```python
from build123d import *

# Parameters (mm, degrees)
F1_DEPTH = 3


with BuildPart() as f1:
    # F0 (on Front) → F1 (new body)
    with BuildSketch(Plane.XZ):
        Polygon((22.4, 25.4), (-25.4, 25.4), (-25.4, -22.4), (-12.7, -22.4), (-12.7, -25.4), (-6.35, -25.4), (-6.35, -22.4), (-1.7526, -22.4), (-1.7526, -18.650325), (-3.96875, -18.650325), (-3.96875, -15.8722), (-1.7526, -15.8722), (-1.7526, -12.6972), (1.7526, -12.6972), (1.7526, -15.8722), (3.96875, -15.8722), (3.96875, -18.650325), (1.7526, -18.650325), (1.7526, -22.4), (6.35, -22.4), (6.35, -25.4), (12.7, -25.4), (12.7, -22.4), (22.4, -22.4), (22.4, -12.7), (25.4, -12.7), (25.4, -6.35), (22.4, -6.35), (22.4, -1.7526), (18.650325, -1.7526), (18.650325, -3.9624), (15.8722, -3.9624), (15.8722, -1.7526), (12.6972, -1.7526), (12.6972, 1.7526), (15.8722, 1.7526), (15.8722, 3.9624), (18.650325, 3.9624), (18.650325, 1.7526), (22.4, 1.7526), (22.4, 6.35), (25.4, 6.35), (25.4, 12.7), (22.4, 12.7), align=None)
    extrude(amount=F1_DEPTH)


solid = f1.part
```
Input: part model. Units: mm. Frame: model coordinates. A direction names the side the tool comes from. Coordinates: 2 decimals unless noted, no trailing zeros. Loops run counter-clockwise (first coordinate to the right, second up) from the corner with the lowest first, then second, coordinate; pieces in that order, holes last. Notation, with made-up numbers: (79.5, 59.25) - (97.5, 59.25) arc R33 ccw to (97.5, 88.25) - close; hole circle Ø4 at (27, 48.25). An arc over 180 degrees is marked (long way). Answer in a Markdown table with one row per item.
(1) Pin query (flat end, axial travel): P1, Ø0.9, axis at x = 24, y = -2, coming from the -Z side; P2, Ø1.5, axis at x = -21.5, y = -2, coming from the -Z side; P3, Ø1.5, axis at y = -1, z = -24.5, coming from the -X side. Return the tip coordinate at first contact, or that it passes through.
Model answer:
| item | result |
|---|---|
| P1 | stops at z = -12.7 |
| P2 | stops at z = -22.4 |
| P3 | stops at x = -12.7 |
(2) Mould query, pull axis X, two halves, no side actions, for faces 5 (the face through (25.4, -1, -10)), 6 (the face through (3, -1, -18.65)), 7 (the face through (0, 0, 0)). Classes: pulls with the +X half, pulls with the -X half, needs draft (parallel to the pull), parting line crosses it, or undercut.
Model answer:
| item | result |
|---|---|
| face 5 | pulls with the +X half |
| face 6 | undercut |
| face 7 | needs draft |
(3) Cut plane C-C on z = 22. Output: boundary loops of the cut face in (x, y), plus the area to 3 significant figures.
Model answer:
| item | result |
|---|---|
| outline | (-25.4, -3) - (22.4, -3) - (22.4, 0) - (-25.4, 0) - close |
| area | 143 mm² |
(4) Cut plane B-B on x = -17.5. Output: boundary loops of the cut face in (y, z).
Model answer:
| item | result |
|---|---|
| outline | (-3, -22.4) - (0, -22.4) - (0, 25.4) - (-3, 25.4) - close |
(5) Cut plane A-A on x = 2.5. Output: boundary loops of the cut face in (y, z).
Model answer:
| item | result |
|---|---|
| outline | (-3, -22.4) - (0, -22.4) - (0, -18.65) - (-3, -18.65) - close; (-3, -15.87) - (0, -15.87) - (0, 25.4) - (-3, 25.4) - close |
(6) Set-up query: faces 1 (the face through (4, -1, -22.4)), 2 (the face through (-19, -1, -22.4)), 3 (the face through (22.4, -1, 19)), 4 (the face through (-3.969, -1, -17)). Return all of +Z, -Z, +X, -X, +Y, -Y with unobstructed straight access to the full face (end or side cutting, diameter ignored); none if empty.
Model answer:
| item | result |
|---|---|
| face 1 | -Z, +Y, -Y |
| face 2 | -Z, -X, +Y, -Y |
| face 3 | +Z, +X, +Y, -Y |
| face 4 | +Y, -Y |
(7) Material intervals for L1, parallel to X at y = -2.3, z = -20; L2, parallel to Z at x = 2, y = -2.3; L3, parallel to X at y = -0.25, z = -17.5, sorted ascending. Write a range as from..to.
Model answer:
| item | result |
|---|---|
| L1 | x = -25.4..-1.75, 1.75..22.4 |
| L2 | z = -22.4..-18.65, -15.87..25.4 |
| L3 | x = -25.4..-3.97, 3.97..22.4 |
